Source: CAD feature listing. Evaluate the final solid. Frame: model axes, mm. Coordinates: 2 decimals unless noted, no trailing zeros. Order: outer loops, then holes, each group sorted by start corner. A loop starts at its lowest first (then second) coordinate and runs counter-clockwise, first axis right, second up. Notation, with made-up numbers: (-20, 21) - (8, 21) arc R13 cw to (8, 29) - close; hole circle Ø6 at (-6, -5). An arc over 180 degrees is marked (long way). One line per question, with ' | ' between items. Start each with the question number.
(1) Contact query for flat-ended pins moving along their axis: P1, Ø4, axis at x = -23.622, y = 0, coming from the -Z side; P2, Ø3.5, axis at x = -23.5, y = 1.5, coming from the -Z side (3 decimals); P3, Ø1, axis at x = 6, y = 2, coming from the +Z side (3 decimals). Output: stop coordinate, or through.
(2) Section D-D (x = -15.5). Return the cut outline in (y, z) (3 decimals), then the cut area to 3 significant figures.
(3) Line query: line 1 along Y through (x, z) = (0, 7.45); line 2 along Y through (x, z) = (0, 2); line 3 along X through (y, z) = (-3, 4.5). Output: solid intervals per line, ascending.
(4) Section A-A (x = 0). Return the cut outline in (y, z) (3 decimals), then the cut area to 3 significant figures.
(5) Section B-B (z = 4.5). Count the separate pieces of the cut face and the enclosed holes in it, then the cut area to 3 significant figures.
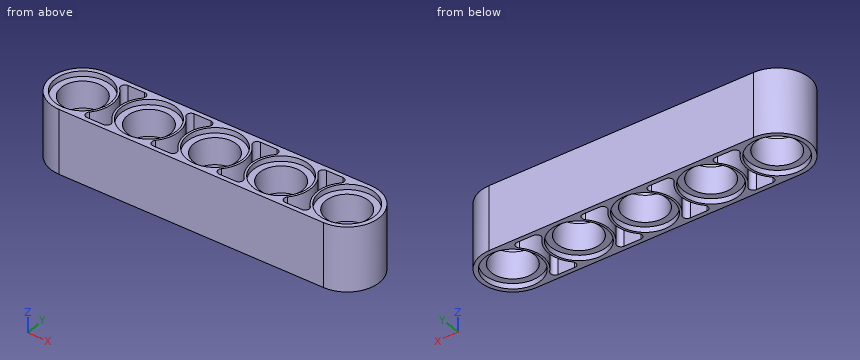
from build123d import *

# Parameters (mm, degrees)
SKETCH1_R           = 3.302
SKETCH1_R_2         = 2.54
BOSS_EXTRUDE1_DEPTH = 3.81
SKETCH1_7_R         = 2.54
BOSS_EXTRUDE2_DEPTH = 3.81
SKETCH2_R           = 3.302
CUT_EXTRUDE1_DEPTH  = 0.635
LPATTERN1_COUNT     = 3
LPATTERN1_PITCH     = 7.874


with BuildPart() as part:
    # Sketch1 → Boss-Extrude1 (new body)
    with BuildSketch(Plane.XY):
        with BuildLine():
            Line((3.937, -3.81), (7.874, -3.81))
            ThreePointArc((7.874, -3.81), (11.684, 0), (7.874, 3.81))
            Line((7.874, 3.81), (3.937, 3.81))
            Line((3.937, 3.81), (3.937, 3.302))
            Line((3.937, 3.302), (4.92278669, 3.302))
            ThreePointArc((4.92278669, 3.302), (5.389414486, 2.994804631), (5.291688354, 2.44475))
            ThreePointArc((5.291688354, 2.44475), (4.318, 0), (5.291688354, -2.44475))
            ThreePointArc((5.291688354, -2.44475), (5.389414486, -2.994804631), (4.92278669, -3.302))
            Line((4.92278669, -3.302), (3.937, -3.302))
            Line((3.937, -3.302), (3.937, -3.81))
        make_face()
        with Locations((7.874, 0)):
            Circle(SKETCH1_R, mode=Mode.SUBTRACT)
        with Locations((7.874, 0)):
            Circle(SKETCH1_R)
        with Locations(Location((7.874, 0, 0), (0, 0, 180))):
            Circle(SKETCH1_R_2, mode=Mode.SUBTRACT)
    extrude(amount=BOSS_EXTRUDE1_DEPTH)


with BuildPart() as body_2:
    # Sketch1_7 → Boss-Extrude2 (new body)
    with BuildSketch(Plane.XY):
        with BuildLine():
            Line((3.937, -3.81), (3.937, -3.302))
            Line((3.937, -3.302), (2.95121331, -3.302))
            ThreePointArc((2.95121331, -3.302), (2.484585514, -2.994804631), (2.582311646, -2.44475))
            ThreePointArc((2.582311646, -2.44475), (3.556, 0), (2.582311646, 2.44475))
            ThreePointArc((2.582311646, 2.44475), (2.484585514, 2.994804631), (2.95121331, 3.302))
            Line((2.95121331, 3.302), (3.937, 3.302))
            Line((3.937, 3.302), (3.937, 3.81))
            Line((3.937, 3.81), (-3.937, 3.81))
            Line((-3.937, 3.81), (-3.937, 3.302))
            Line((-3.937, 3.302), (-2.95121331, 3.302))
            ThreePointArc((-2.95121331, 3.302), (-2.484585514, 2.994804631), (-2.582311646, 2.44475))
            ThreePointArc((-2.582311646, 2.44475), (-3.556, 0), (-2.582311646, -2.44475))
            ThreePointArc((-2.582311646, -2.44475), (-2.484585514, -2.994804631), (-2.95121331, -3.302))
            Line((-2.95121331, -3.302), (-3.937, -3.302))
            Line((-3.937, -3.302), (-3.937, -3.81))
            Line((-3.937, -3.81), (3.937, -3.81))
        make_face()
        with Locations(Location((0, 0, 0), (0, 0, 180))):
            Circle(SKETCH1_7_R, mode=Mode.SUBTRACT)
    boss_extrude2 = extrude(amount=BOSS_EXTRUDE2_DEPTH)


with BuildPart() as cut_extrude1_tool:
    # Sketch2 → Cut-Extrude1 (new body)
    with BuildSketch(Plane.XY):
        with Locations((7.874, 0)):
            Circle(SKETCH2_R)
        Circle(SKETCH2_R)
    cut_extrude1 = extrude(amount=CUT_EXTRUDE1_DEPTH)


with BuildPart() as part_1:
    add(part.part)

    # Cut-Extrude1: cut by cut_extrude1_tool
    add(cut_extrude1_tool.part, mode=Mode.SUBTRACT)


with BuildPart() as body_2_1:
    add(body_2.part)

    # Cut-Extrude1: cut by cut_extrude1_tool
    add(cut_extrude1_tool.part, mode=Mode.SUBTRACT)

    # LPattern1: Boss-Extrude2, Cut-Extrude1 ×3
    with Locations(*[(-i * LPATTERN1_PITCH, 0, 0) for i in range(1, LPATTERN1_COUNT)]):
        add(boss_extrude2)
        add(cut_extrude1, mode=Mode.SUBTRACT)


with BuildPart() as body_3:
    # Mirror2: mirrored copy
    add(part_1.part.mirror(Plane(origin=(-7.874, 0, 0), x_dir=(0, 0, 1), z_dir=(1, 0, 0))))


with BuildPart() as part_2:
    add(part_1.part)

    # Combine1: union body 3, body 2
    add(body_3.part)
    add(body_2_1.part)

    # Mirror3: part across plane


with BuildPart() as part_3:
    add(part_2.part)
    add(part_2.part.mirror(Plane.XY.offset(3.81)))


solid = part_3.part
Response values:
1) P1: passes through | P2: stops at z = 0.635 | P3: stops at z = 6.985
2) outline: (-3.81, 0) - (-3.293, 0) - (-3.293, 0.635) - (-2.528, 0.635) - (-2.528, 6.985) - (-3.293, 6.985) - (-3.293, 7.62) - (-3.81, 7.62) - close; (2.528, 0.635) - (3.293, 0.635) - (3.293, 0) - (3.81, 0) - (3.81, 7.62) - (3.293, 7.62) - (3.293, 6.985) - (2.528, 6.985) - close | area: 17.6 mm²
3) line 1: y = -3.81 to -3.3, 3.3 to 3.81 | line 2: y = -3.81 to -2.54, 2.54 to 3.81 | line 3: x = -25.97 to -21.14, -18.23 to -13.26, -10.36 to -5.39, -2.49 to 2.49, 5.39 to 10.22
4) outline: (-3.81, 0) - (-3.302, 0) - (-3.302, 0.635) - (-2.54, 0.635) - (-2.54, 6.985) - (-3.302, 6.985) - (-3.302, 7.62) - (-3.81, 7.62) - close; (2.54, 0.635) - (3.302, 0.635) - (3.302, 0) - (3.81, 0) - (3.81, 7.62) - (3.302, 7.62) - (3.302, 6.985) - (2.54, 6.985) - close | area: 17.4 mm²
5) separate pieces: 1 | enclosed holes: 9 | area: 138 mm²
